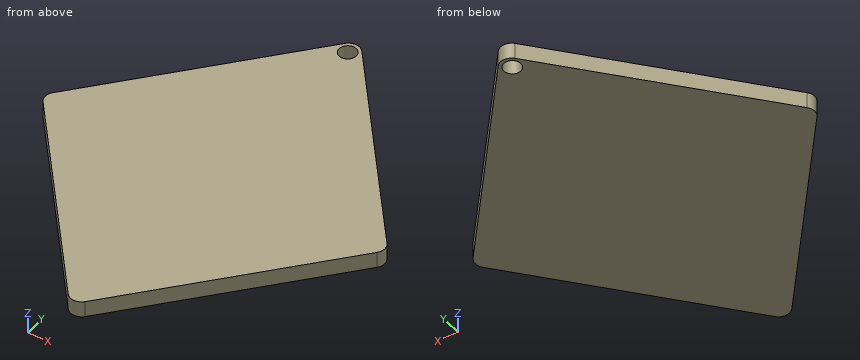
```python
from build123d import *

# Parameters (mm, degrees)
F0_R     = 3.40817912
F1_DEPTH = 6.35


# Not quite as in the source:
# - a length typed as a fraction of an inch, garbled in the dataset ("3 / 203.2 mm" for 3/8 in), is restored


with BuildPart() as f1:
    # F0 (on Top) → F1 (new body)
    with BuildSketch(Plane.XY):
        with BuildLine():
            ThreePointArc((3.4050675497, 78.4919985147), (0, 80.0798075896), (-3.4050675497, 78.4919985147))
            Line((-3.4050675497, 78.4919985147), (-66.8702067023, 2.8571909251))
            ThreePointArc((-66.8702067023, 2.8571909251), (-67.9101391526, 0), (-66.8702067023, -2.8571909251))
            Line((-66.8702067023, -2.8571909251), (-3.4050675497, -78.4919985147))
            ThreePointArc((-3.4050675497, -78.4919985147), (0, -80.0798075896), (3.4050675497, -78.4919985147))
            Line((3.4050675497, -78.4919985147), (66.8702067023, -2.8571909251))
            ThreePointArc((66.8702067023, -2.8571909251), (67.9101391526, 0), (66.8702067023, 2.8571909251))
            Line((66.8702067023, 2.8571909251), (3.4050675497, 78.4919985147))
        make_face()
        with Locations((0, 75.311)):
            Circle(F0_R, mode=Mode.SUBTRACT)
    extrude(amount=F1_DEPTH)


solid = f1.part
```
Geometry: final body of the model. Coordinates: model frame, mm. Coordinates: 2 decimals unless noted, no trailing zeros. Order: outer loops, then holes, each group sorted by start corner. A loop starts at its lowest first (then second) coordinate and runs counter-clockwise, first axis right, second up.
Item 1: Section query D-D (x = -31). Output: boundary loops of the cut face in (y, z), then the cut area to 3 significant figures.
Answer:
outline: (-45.61, 0) - (45.61, 0) - (45.61, 6.35) - (-45.61, 6.35) - close
area: 579 mm2
Item 2: Contact query for flat-ended pins moving along their axis: P1, Ø1.5, axis at y = 22, z = 1.5, coming from the +X side; P2, Ø1.5, axis at y = -57, z = 2, coming from the +X side; P3, Ø2, axis at x = 43.5, z = 3, coming from the +Y side. Output: stop coordinate, or through.
Answer:
P1: stops at x = 51.44
P2: stops at x = 22.07
P3: stops at y = 31.9
Item 3: Section query B-B (z = 2.75). Output: boundary loops of the cut face in (x, y) (3 decimals).
Answer:
outline: (-66.87, -2.857) - (-3.405, -78.492) arc R4.445 ccw to (3.405, -78.492) - (66.87, -2.857) arc R4.445 ccw to (66.87, 2.857) - (3.405, 78.492) arc R4.445 ccw to (-3.405, 78.492) - (-66.87, 2.857) arc R4.445 ccw to start; hole circle Ø6.816 at (0, 75.311)
Item 4: Section query C-C (y = -38). Output: boundary loops of the cut face in (x, z), then the cut area to 3 significant figures.
Answer:
outline: (-37.38, 0) - (37.38, 0) - (37.38, 6.35) - (-37.38, 6.35) - close
area: 475 mm2
Item 5: Material intervals for line 1 along Y through (x, z) = (1.5, 1.75); line 2 along Y through (x, z) = (-59, 4.5); line 3 along X through (y, z) = (-45.5, 1.5), sorted ascending.
Answer:
line 1: y = -79.82 to 72.25, 78.37 to 79.82
line 2: y = -12.24 to 12.24
line 3: x = -31.09 to 31.09
Item 6: Section query A-A (x = 0). Output: boundary loops of the cut face in (y, z).
Answer:
outline: (-80.08, 0) - (71.9, 0) - (71.9, 6.35) - (-80.08, 6.35) - close; (78.72, 0) - (80.08, 0) - (80.08, 6.35) - (78.72, 6.35) - close
